For this review, take the finished solid that the model builds, in its own axes (mm). Face numbers are marked on the shaded views. A direction names the side the tool comes from. Give positions to 0.01 mm unless a question says otherwise; leave off trailing zeros. Write each loop counter-clockwise with the first axis right and the second up, starting at its lowest first coordinate (ties: lowest second). Pieces come first, ordered by that corner, then holes.
Q1. Mouldability with a two-part tool opening along Y and no side actions: class the marked faces 1, 2 and 3 as released by +Y, released by -Y, zero draft, split by the parting line, or undercut.
Q2. Insertion check: P1, Ø1, axis at x = 1.5, y = -1, coming from the +Z side; P2, Ø1.5, axis at x = 2, z = -1, coming from the -Y side. Each pin has a flat end and moves straight along its axis. Give the tip position at first contact, or say it passes through.
Q3. Machinability: for the marked faces 4 and 5, which of the approach directions +Z, -Z, +X, -X, +Y, -Y give a long, thin tool a straight path to every point of the face, cutting with its end or side? Answer none if there is none.
Q4. We need section C-C (x = 1.05). Write out the cut boundary in (y, z), then the cut area to 3 significant figures.
Q5. We need section A-A (z = 0). Write out the cut boundary in (x, y).
Q6. We need section D-D (z = -3.25). Write out the cut boundary in (x, y), then the cut area to 3 significant figures.
Q7. For line 1 (Y direction, x = 1.9, z = 0); line 2 (Y direction, x = 2.35, z = 0); line 3 (X direction, y = 0.75, z = -4.25), list the stretches that pass through material, from the lowest coordinate up.
```python
from build123d import *

# Parameters (mm, degrees)
SKETCH1_R           = 5.5
BOSS_EXTRUDE1_DEPTH = 2
SKETCH2_R           = 3.8
BOSS_EXTRUDE2_DEPTH = 1
SKETCH3_R           = 1.8
CUT_EXTRUDE1_DEPTH  = 20


with BuildPart() as part:
    # Sketch1 → Boss-Extrude1 (new body)
    with BuildSketch(Plane(origin=(0, 0, 0), x_dir=(0, 0, -1), z_dir=(1, 0, 0))):
        Circle(SKETCH1_R)
    extrude(amount=BOSS_EXTRUDE1_DEPTH)

    # Sketch2 → Boss-Extrude2 (add)
    with BuildSketch(Plane(origin=(2, 0, 0), x_dir=(0, 0, -1), z_dir=(1, 0, 0))):
        Circle(SKETCH2_R)
    extrude(amount=BOSS_EXTRUDE2_DEPTH)

    # Sketch3 → Cut-Extrude1 (cut)
    with BuildSketch(Plane.ZY):
        Circle(SKETCH3_R)
    extrude(amount=-CUT_EXTRUDE1_DEPTH, mode=Mode.SUBTRACT)


solid = part.part
```
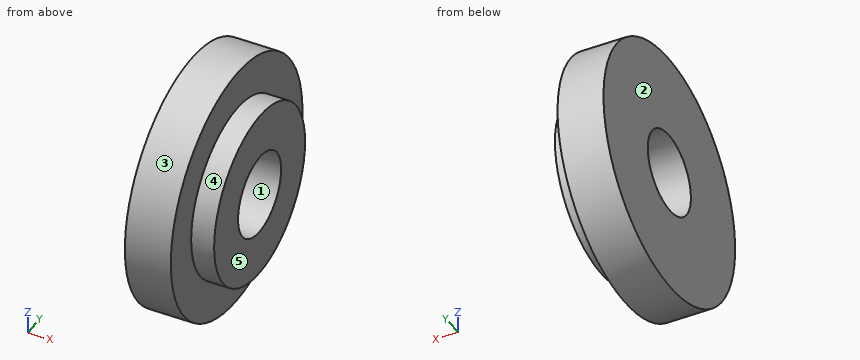
Computed:
1. face 1: undercut
1. face 2: zero draft
1. face 3: split by the parting line
2. P1: stops at z = 5.48
2. P2: stops at y = -5.49
3. face 4: +X
3. face 5: +Z, -Z, +X, +Y, -Y
4. outline: circle Ø11 at (0, 0); hole circle Ø3.6 at (0, 0)
4. area: 84.9 mm2
5. outline: (0, -5.5) - (2, -5.5) - (2, -3.8) - (3, -3.8) - (3, -1.8) - (0, -1.8) - close; (0, 1.8) - (3, 1.8) - (3, 3.8) - (2, 3.8) - (2, 5.5) - (0, 5.5) - close
6. outline: (0, -4.44) - (2, -4.44) - (2, -1.97) - (3, -1.97) - (3, 1.97) - (2, 1.97) - (2, 4.44) - (0, 4.44) - close
6. area: 21.7 mm2
7. line 1: y = -5.5 to -1.8, 1.8 to 5.5
7. line 2: y = -3.8 to -1.8, 1.8 to 3.8
7. line 3: x = 0 to 2
